```python
from build123d import *

# Parameters (mm, degrees)
F3_DEPTH = 0.5
F4_COUNT = 5


# Not quite as in the source:
# - a feature names something its author has since deleted; it is built from what else it names


with BuildPart() as f1:
    # F0 (on Front) → F1 (revolve)
    with BuildSketch(Plane.XZ):
        with BuildLine():
            Line((0, 9.0353097767), (0, 0))
            Line((0, 0), (10, 0))
            Line((10, 0), (10, 2))
            Line((10, 2), (9, 2))
            ThreePointArc((9, 2), (9.2928932188, 2.7071067812), (10, 3))
            add(Edge.make_bspline(
                [(10, 3), (5.8599692942, 7.1514955665), (3.7520111059, 12.6606088045), (2.9057694535, 18.3767723616)],
                knots=[0, 0, 0, 0, 0.2723692437, 0.2723692437, 0.2723692437, 0.2723692437], degree=3))
            Line((2.9057694535, 18.3767723616), (1.4480197044, 17.810525763))
            Line((1.4480197044, 17.810525763), (2.4403755087, 11.1617380753))
            Line((2.4403755087, 11.1617380753), (0, 9.0353097767))
        make_face()
        with BuildLine():
            Line((0, 51), (0, 44))
            add(Edge.make_bspline(
                [(1.7302031744, 44.8584092014), (1.2074659957, 44.6052050311), (0.6322180551, 44.3196864642), (0, 44)],
                knots=[0.9786462718, 0.9786462718, 0.9786462718, 0.9786462718, 1, 1, 1, 1], degree=3))
            Line((1.7302031744, 44.8584092014), (3.7866074126, 49.6094115078))
            Line((3.7866074126, 49.6094115078), (0, 51))
        make_face()
        with BuildLine():
            Line((1.1113585206, 20.0661569834), (1.4480197044, 17.810525763))
            Line((1.4480197044, 17.810525763), (2.9057694535, 18.3767723616))
            add(Edge.make_bspline(
                [(2.9057694535, 18.3767723616), (2.7448272283, 19.4638992829), (2.6295215739, 20.5585152608), (2.554553193, 21.6527055151)],
                knots=[0.2723692437, 0.2723692437, 0.2723692437, 0.2723692437, 0.32416971, 0.32416971, 0.32416971, 0.32416971], degree=3))
            Line((2.554553193, 21.6527055151), (1.1113585206, 21.8489095134))
            Line((1.1113585206, 21.8489095134), (1.1113585206, 20.0661569834))
        make_face()
        with BuildLine():
            add(Edge.make_bspline(
                [(2.9057694535, 18.3767723616), (2.7448272283, 19.4638992829), (2.6295215739, 20.5585152608), (2.554553193, 21.6527055151)],
                knots=[0.2723692437, 0.2723692437, 0.2723692437, 0.2723692437, 0.32416971, 0.32416971, 0.32416971, 0.32416971], degree=3))
            Line((2.9057694535, 18.3767723616), (9.0618459508, 20.7680314779))
            Line((9.0618459508, 20.7680314779), (2.554553193, 21.6527055151))
        make_face()
        with BuildLine():
            Line((0, 44), (0, 41.3304418325))
            Line((0, 41.3304418325), (2.4403755087, 41.3304418325))
            Line((2.4403755087, 41.3304418325), (1.1113585206, 31.4957089722))
            Line((1.1113585206, 31.4957089722), (1.1113585206, 21.8489095134))
            Line((1.1113585206, 21.8489095134), (2.554553193, 21.6527055151))
            add(Edge.make_bspline(
                [(2.554553193, 21.6527055151), (1.9701230673, 30.1826716243), (4.9959561324, 43.9653621083), (7.8662442935, 47.8305934345), (1.7302031744, 44.8584092014)],
                knots=[0.32416971, 0.32416971, 0.32416971, 0.32416971, 0.727989996, 0.9786462718, 0.9786462718, 0.9786462718, 0.9786462718], degree=3))
            add(Edge.make_bspline(
                [(1.7302031744, 44.8584092014), (1.2074659957, 44.6052050311), (0.6322180551, 44.3196864642), (0, 44)],
                knots=[0.9786462718, 0.9786462718, 0.9786462718, 0.9786462718, 1, 1, 1, 1], degree=3))
        make_face()
    revolve(axis=Axis((0, 0, 22), (0, 0, 1)))



with BuildPart() as f3:
    # F2 (on Front) → F3 (new body, symmetric)
    with BuildSketch(Plane.XZ):
        Polygon((-0.3592191799, 51.9545889315), (-0.3592191799, 50.8362587973), (3.4741000272, 49.5302081108), align=None)
    extrude(amount=F3_DEPTH, both=True)


with BuildPart() as f1_1:
    add(f1.part)

    add(f3.part)  # F4 merges F3
    # F4: F3 ×5 about axis
    f4_axis = Axis((0, 0, 47.5), (0, 0, 1))
    for i in range(1, F4_COUNT):
        add(f3.part.rotate(f4_axis, i * 360 / F4_COUNT))


solid = f1_1.part
```
Source: CAD feature listing. Evaluate the final solid. Frame: model axes, mm. A direction names the side the tool comes from. Round coordinates to 2 decimals unless told otherwise and drop trailing zeros. Use CSV: the item, a comma, the result in double quotes.
Q1. Reachability of faces 1 (the conical face through (-0.301, 2.296, 46.211)), 2 (the conical face through (-0.286, -1.288, 50.515)) from +Z, -Z, +X, -X, +Y, -Y: full face, straight path, thin tool, end or side. Return the list, or none.
Reported:
face 1,"none"
face 2,"+Z"
Q2. Section query A-A, the plane y = -4.5. Give the number of separate pieces and of enclosed holes in the cut face, then the cut area to 3 significant figures.
Reported:
separate pieces,"3"
enclosed holes,"0"
area,"200 mm^2"
Q3. Mould query, pull axis X, two halves, no side actions, for faces 3 (the conical face through (3.139, 0.988, 18.526)), 4 (the cylindrical face through (-0.88, -0.68, 25.7)), 5 (the flat face through (0.513, -1.601, 50.664)), 6 (the conical face through (0.372, 0.117, 9.375)). Classes: pulls with the +X half, pulls with the -X half, needs draft (parallel to the pull), parting line crosses it, or undercut.
Reported:
face 3,"parting line crosses it"
face 4,"undercut"
face 5,"pulls with the +X half"
face 6,"undercut"
Q4. Pin query (flat end, axial travel): pin 1 Ø8 at (x, z) = (-0.5, 40) entering from +Y; pin 2 Ø1.1 at (x, z) = (2, 51) entering from -Y; pin 3 Ø10 at (x, y) = (6.5, 4.5) entering from -Z; pin 4 Ø8 at (y, z) = (-4, 31) entering from +X. Return the tip coordinate at first contact, or that it passes through.
Reported:
pin 1,"y = 5.87"
pin 2,"y = -0.5"
pin 3,"z = 0"
pin 4,"x = 3.01"
Q5. Ray query, line 1 along X through (y, z) = (-0.25, 10); line 2 along Z through (x, y) = (-5.5, 2.75); line 3 along Z through (x, y) = (3, -8.75). Return the intervals inside material, ascending.
Reported:
line 1,"-5.26 to -1.08, 1.08 to 5.26"
line 2,"0 to 8.2, 19.64 to 21.16, 44.69 to 46.47"
line 3,"0 to 2, 2.66 to 3.79"
